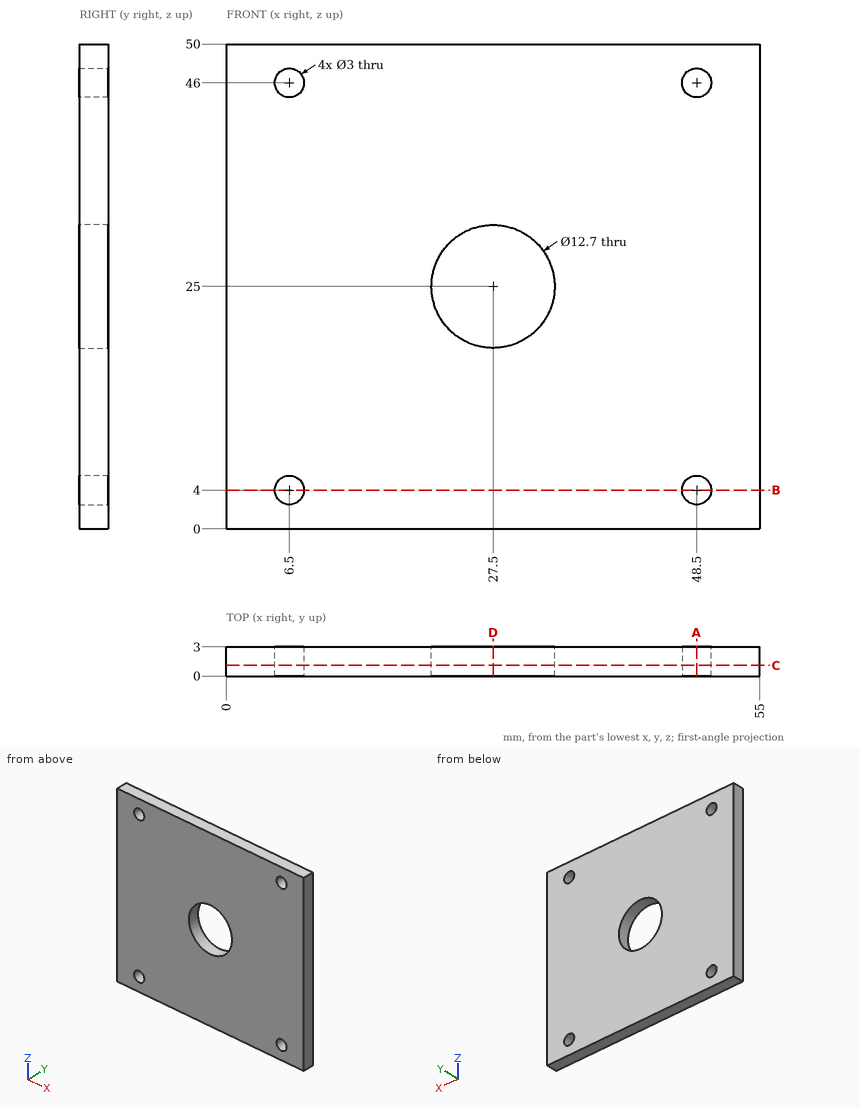
Study the drawing (mm; zero at the part's minimum x, y, z) and answer. Give positions to 0.01 mm unless a question says otherwise; leave off trailing zeros. Write each loop counter-clockwise with the first axis right and the second up, starting at its lowest first coordinate (ties: lowest second). Pieces come first, ordered by that corner, then holes. Notation, with made-up numbers: (-35, 10.5) - (18, 10.5) arc R7 ccw to (18, 21.5) - close; hole circle Ø6 at (70, 51.5). An arc over 180 degrees is marked (long way). Use CSV: the item, a comma, the result in double quotes. Start each with the question number.
(1) Find section D-D (x = 27.5). Give the vertices of the cut face in (y, z), plus the area to 3 significant figures.
(2) Find section B-B (z = 4). Give the vertices of the cut face in (x, y).
(3) Consider line 1 along Z through (x, y) = (48.5, 1.3); line 2 along X through (y, z) = (2.25, 46); line 3 along Z through (x, y) = (48, 1.8). Determine where each line is inside the solid, lowest interval first.
(4) Find section C-C (y = 1.1). Give the vertices of the cut face in (x, z), plus the area to 3 significant figures.
(5) Find section A-A (x = 48.5). Give the vertices of the cut face in (y, z).
Findings below:
1,outline,"(0, 0) - (3, 0) - (3, 18.65) - (0, 18.65) - close; (0, 31.35) - (3, 31.35) - (3, 50) - (0, 50) - close"
1,area,"112 mm2"
2,outline,"(0, 0) - (5, 0) - (5, 3) - (0, 3) - close; (8, 0) - (47, 0) - (47, 3) - (8, 3) - close; (50, 0) - (55, 0) - (55, 3) - (50, 3) - close"
3,line 1,"0 to 2.5, 5.5 to 44.5, 47.5 to 50"
3,line 2,"0 to 5, 8 to 47, 50 to 55"
3,line 3,"0 to 2.59, 5.41 to 44.59, 47.41 to 50"
4,outline,"(0, 0) - (55, 0) - (55, 50) - (0, 50) - close; hole circle Ø3 at (6.5, 4); hole circle Ø3 at (6.5, 46); hole circle Ø12.7 at (27.5, 25); hole circle Ø3 at (48.5, 4); hole circle Ø3 at (48.5, 46)"
4,area,"2,600 mm2"
5,outline,"(0, 0) - (3, 0) - (3, 2.5) - (0, 2.5) - close; (0, 5.5) - (3, 5.5) - (3, 44.5) - (0, 44.5) - close; (0, 47.5) - (3, 47.5) - (3, 50) - (0, 50) - close"
